Read the model definition and answer for the solid it produces. Units are mm, in the model's axes. Face numbers are marked on the shaded views. A direction names the side the tool comes from. Coordinates: 2 decimals unless noted, no trailing zeros. Write each loop counter-clockwise with the first axis right and the second up, starting at its lowest first coordinate (ties: lowest second). Pieces come first, ordered by that corner, then holes.
1) The part is cut by section B-B (x = 181.5). Determine the outline of the cut face in (y, z), then the cut area to 3 significant figures.
2) Which of the six approach directions +Z, -Z, +X, -X, +Y, -Y give full straight-line access (tool end or side, diameter ignored) to the marked faces 1, 2 and 3?
3) Find the intervals of material crossed by line 1 (Y direction, x = 63.5, z = 29); line 2 (X direction, y = 35, z = 9); line 3 (X direction, y = -31, z = -28.5), in increasing order.
4) The part is cut by section A-A (x = 71). Determine the outline of the cut face in (y, z), then the cut area to 3 significant figures.
5) Determine the mould class of the marked faces 4, 5 and 6 for opening direction X: +X half, -X half, draft (parallel to the pull), parting line (faces both ways), or undercut.
6) Each of these flat-tipped pins is pushed along its axis until it touches: pin 1 Ø2 at (x, y) = (318.5, -4.5) entering from -Z; pin 2 Ø1.5 at (x, z) = (123, -9.5) entering from +Y; pin 3 Ø5.5 at (x, y) = (256.5, -12.5) entering from -Z. Where does it stop, or does it pass through?
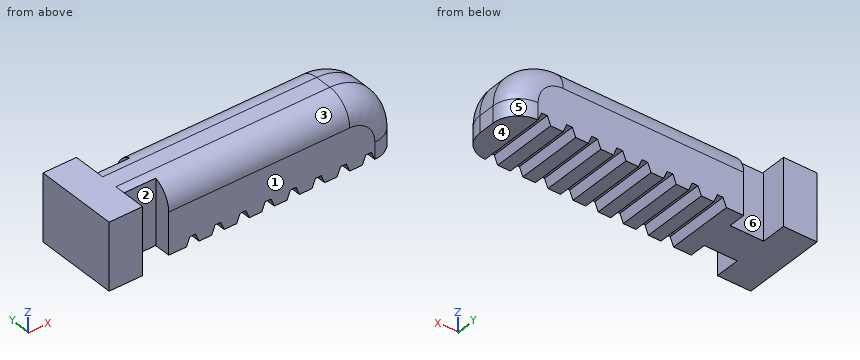
from build123d import *

# Parameters (mm, degrees)
BOSS_EXTRUDE1_DEPTH          = 40
FILLET1_R                    = 60
FILLET2_R                    = 30
SKETCH3_W                    = 15
SKETCH3_H                    = 109.922704731
CUT_EXTRUDE1_DEPTH           = 10
CUT_EXTRUDE1_DRAFT           = -22
CUT_EXTRUDE1_PROFILE_2_DEPTH = 10
CUT_EXTRUDE1_PROFILE_2_DRAFT = -22
CUT_EXTRUDE1_PROFILE_3_DEPTH = 10
CUT_EXTRUDE1_PROFILE_3_DRAFT = -22
CUT_EXTRUDE1_PROFILE_4_DEPTH = 10
CUT_EXTRUDE1_PROFILE_4_DRAFT = -22
CUT_EXTRUDE1_PROFILE_5_DEPTH = 10
CUT_EXTRUDE1_PROFILE_5_DRAFT = -22
CUT_EXTRUDE1_PROFILE_6_DEPTH = 10
CUT_EXTRUDE1_PROFILE_6_DRAFT = -22
CUT_EXTRUDE1_PROFILE_7_DEPTH = 10
CUT_EXTRUDE1_PROFILE_7_DRAFT = -22
CUT_EXTRUDE1_PROFILE_8_DEPTH = 10
CUT_EXTRUDE1_PROFILE_8_DRAFT = -22


with BuildPart() as part:
    # Sketch1 → Boss-Extrude1 (new, symmetric)
    with BuildSketch(Plane.XY):
        Polygon((0, 41.520471033), (0, -58.474576271), (40, -58.474576271), (40, -28.474576271), (79.370562847, -28.474576271), (79.370562847, -48.090018927), (355.561633386, -48.090018927), (355.561633386, -28.474576271), (355.561633386, 11.525423729), (355.561633386, 31.909981073), (80, 31.909981073), (80, 11.520471033), (40, 11.520471033), (40, 41.520471033), align=None)
    extrude(amount=BOSS_EXTRUDE1_DEPTH, both=True)

    # Fillet1
    fillet1_edges = [part.edges().sort_by_distance(p)[0] for p in [
        (355.561633386, -8.090018927, 40),
    ]]
    fillet(fillet1_edges, radius=FILLET1_R)

    # Fillet2
    # the kernel refuses this fillet: 30 mm, written as the material it takes off along each edge
    with BuildSketch(Plane(origin=(355.561633386, -48.090018927, -115), x_dir=(0, 1, 0), z_dir=(0, 0, 1)), Plane(origin=(355.561633386, 31.909981073, -115), x_dir=(-1, 0, 0), z_dir=(0, 0, 1))) as fillet2_piece_1:
        with BuildLine():
            CenterArc((FILLET2_R, FILLET2_R), FILLET2_R, 180, 90)
            Line((0, FILLET2_R), (0, 0))
            Line((0, 0), (FILLET2_R, 0))
        make_face()
    extrude(amount=95, mode=Mode.SUBTRACT)
    with BuildSketch(Plane(origin=(295.561633386, -48.090018927, -20), x_dir=(1, 0, 0), z_dir=(0, 0, -1))) as fillet2_piece_2:
        with BuildLine():
            CenterArc((60 - FILLET2_R, -FILLET2_R), FILLET2_R, 0, 90)
            Line((60 - FILLET2_R, 0), (60, 0))
            Line((60, 0), (60, -FILLET2_R))
        make_face()
    revolve(axis=Axis((295.561633386, -48.090018927, -20), (0, -1, 0)), revolution_arc=90, mode=Mode.SUBTRACT)
    with BuildSketch(Plane(origin=(295.561633386, 31.909981073, -20), x_dir=(1, 0, 0), z_dir=(0, 0, -1))) as fillet2_piece_3:
        with BuildLine():
            CenterArc((60 - FILLET2_R, FILLET2_R), FILLET2_R, 270, 90)
            Line((60, FILLET2_R), (60, 0))
            Line((60, 0), (60 - FILLET2_R, 0))
        make_face()
    revolve(axis=Axis((295.561633386, 31.909981073, -20), (0, -1, 0)), revolution_arc=90, mode=Mode.SUBTRACT)
    with BuildSketch(Plane(origin=(4.370562847, -48.090018927, 40), x_dir=(0, 1, 0), z_dir=(1, 0, 0))) as fillet2_piece_4_section:
        with BuildLine():
            CenterArc((FILLET2_R, -FILLET2_R), FILLET2_R, 90, 90)
            Line((0, -FILLET2_R), (0, 0))
            Line((0, 0), (FILLET2_R, 0))
        make_face()
    fillet2_piece_4 = extrude(amount=291.191070539, mode=Mode.PRIVATE)
    fillet2_piece_4 = split(fillet2_piece_4, bisect_by=Plane(origin=(40, -25.894757841, 39.446684124), z_dir=(1, 0, 0)), keep=Keep.TOP, mode=Mode.PRIVATE)
    add(fillet2_piece_4, mode=Mode.SUBTRACT)
    with BuildSketch(Plane(origin=(295.561633386, 31.909981073, 40), x_dir=(0, 0, -1), z_dir=(-1, 0, 0))) as fillet2_piece_5_section:
        with BuildLine():
            CenterArc((FILLET2_R, FILLET2_R), FILLET2_R, 180, 90)
            Line((0, FILLET2_R), (0, 0))
            Line((0, 0), (FILLET2_R, 0))
        make_face()
    fillet2_piece_5 = extrude(amount=290.561633386, mode=Mode.PRIVATE)
    fillet2_piece_5 = split(fillet2_piece_5, bisect_by=Plane(origin=(40, 26.935715602, 30.794780606), z_dir=(1, 0, 0)), keep=Keep.TOP, mode=Mode.PRIVATE)
    add(fillet2_piece_5, mode=Mode.SUBTRACT)


with BuildPart() as cut_extrude1_tool:
    # Sketch3 → Cut-Extrude1 (with draft: the straight prism first)
    with BuildSketch(Plane(origin=(0, 0, -40), x_dir=(-1, 0, 0), z_dir=(0, 0, -1))):
        with Locations((-318.061633386, -9.051561529)):
            Rectangle(SKETCH3_W, SKETCH3_H)
    extrude(amount=-CUT_EXTRUDE1_DEPTH)
    # Cut-Extrude1: the draft: its side faces are tilted about the plane it starts from
    cut_extrude1_sides = [cut_extrude1_tool.faces().sort_by_distance(p)[0] for p in [
        (325.561633386, -9.051561529, -35),
        (318.061633386, -64.012913894, -35),
        (310.561633386, -9.051561529, -35),
        (318.061633386, 45.909790837, -35),
    ]]
    draft(cut_extrude1_sides, Plane(origin=(0, 0, -40), x_dir=(-1, 0, 0), z_dir=(0, 0, -1)), CUT_EXTRUDE1_DRAFT)


with BuildPart() as part_1:
    add(part.part)

    # Cut-Extrude1: cut by cut_extrude1_tool
    add(cut_extrude1_tool.part, mode=Mode.SUBTRACT)


with BuildPart() as cut_extrude1_profile_2_tool:
    # Sketch3 → Cut-Extrude1 profile 2 (with draft: the straight prism first)
    with BuildSketch(Plane(origin=(0, 0, -40), x_dir=(-1, 0, 0), z_dir=(0, 0, -1))):
        with Locations((-288.061633386, -9.051561529)):
            Rectangle(SKETCH3_W, SKETCH3_H)
    extrude(amount=-CUT_EXTRUDE1_PROFILE_2_DEPTH)
    # Cut-Extrude1 profile 2: the draft: its side faces are tilted about the plane it starts from
    cut_extrude1_profile_2_sides = [cut_extrude1_profile_2_tool.faces().sort_by_distance(p)[0] for p in [
        (295.561633386, -9.051561529, -35),
        (288.061633386, -64.012913894, -35),
        (280.561633386, -9.051561529, -35),
        (288.061633386, 45.909790837, -35),
    ]]
    draft(cut_extrude1_profile_2_sides, Plane(origin=(0, 0, -40), x_dir=(-1, 0, 0), z_dir=(0, 0, -1)), CUT_EXTRUDE1_PROFILE_2_DRAFT)


with BuildPart() as part_2:
    add(part_1.part)

    # Cut-Extrude1 profile 2: cut by cut_extrude1_profile_2_tool
    add(cut_extrude1_profile_2_tool.part, mode=Mode.SUBTRACT)


with BuildPart() as cut_extrude1_profile_3_tool:
    # Sketch3 → Cut-Extrude1 profile 3 (with draft: the straight prism first)
    with BuildSketch(Plane(origin=(0, 0, -40), x_dir=(-1, 0, 0), z_dir=(0, 0, -1))):
        with Locations((-258.061633386, -9.051561529)):
            Rectangle(SKETCH3_W, SKETCH3_H)
    extrude(amount=-CUT_EXTRUDE1_PROFILE_3_DEPTH)
    # Cut-Extrude1 profile 3: the draft: its side faces are tilted about the plane it starts from
    cut_extrude1_profile_3_sides = [cut_extrude1_profile_3_tool.faces().sort_by_distance(p)[0] for p in [
        (265.561633386, -9.051561529, -35),
        (258.061633386, -64.012913894, -35),
        (250.561633386, -9.051561529, -35),
        (258.061633386, 45.909790837, -35),
    ]]
    draft(cut_extrude1_profile_3_sides, Plane(origin=(0, 0, -40), x_dir=(-1, 0, 0), z_dir=(0, 0, -1)), CUT_EXTRUDE1_PROFILE_3_DRAFT)


with BuildPart() as part_3:
    add(part_2.part)

    # Cut-Extrude1 profile 3: cut by cut_extrude1_profile_3_tool
    add(cut_extrude1_profile_3_tool.part, mode=Mode.SUBTRACT)


with BuildPart() as cut_extrude1_profile_4_tool:
    # Sketch3 → Cut-Extrude1 profile 4 (with draft: the straight prism first)
    with BuildSketch(Plane(origin=(0, 0, -40), x_dir=(-1, 0, 0), z_dir=(0, 0, -1))):
        with Locations((-228.061633386, -9.051561529)):
            Rectangle(SKETCH3_W, SKETCH3_H)
    extrude(amount=-CUT_EXTRUDE1_PROFILE_4_DEPTH)
    # Cut-Extrude1 profile 4: the draft: its side faces are tilted about the plane it starts from
    cut_extrude1_profile_4_sides = [cut_extrude1_profile_4_tool.faces().sort_by_distance(p)[0] for p in [
        (235.561633386, -9.051561529, -35),
        (228.061633386, -64.012913894, -35),
        (220.561633386, -9.051561529, -35),
        (228.061633386, 45.909790837, -35),
    ]]
    draft(cut_extrude1_profile_4_sides, Plane(origin=(0, 0, -40), x_dir=(-1, 0, 0), z_dir=(0, 0, -1)), CUT_EXTRUDE1_PROFILE_4_DRAFT)


with BuildPart() as part_4:
    add(part_3.part)

    # Cut-Extrude1 profile 4: cut by cut_extrude1_profile_4_tool
    add(cut_extrude1_profile_4_tool.part, mode=Mode.SUBTRACT)


with BuildPart() as cut_extrude1_profile_5_tool:
    # Sketch3 → Cut-Extrude1 profile 5 (with draft: the straight prism first)
    with BuildSketch(Plane(origin=(0, 0, -40), x_dir=(-1, 0, 0), z_dir=(0, 0, -1))):
        with Locations((-198.061633386, -9.051561529)):
            Rectangle(SKETCH3_W, SKETCH3_H)
    extrude(amount=-CUT_EXTRUDE1_PROFILE_5_DEPTH)
    # Cut-Extrude1 profile 5: the draft: its side faces are tilted about the plane it starts from
    cut_extrude1_profile_5_sides = [cut_extrude1_profile_5_tool.faces().sort_by_distance(p)[0] for p in [
        (205.561633386, -9.051561529, -35),
        (198.061633386, -64.012913894, -35),
        (190.561633386, -9.051561529, -35),
        (198.061633386, 45.909790837, -35),
    ]]
    draft(cut_extrude1_profile_5_sides, Plane(origin=(0, 0, -40), x_dir=(-1, 0, 0), z_dir=(0, 0, -1)), CUT_EXTRUDE1_PROFILE_5_DRAFT)


with BuildPart() as part_5:
    add(part_4.part)

    # Cut-Extrude1 profile 5: cut by cut_extrude1_profile_5_tool
    add(cut_extrude1_profile_5_tool.part, mode=Mode.SUBTRACT)


with BuildPart() as cut_extrude1_profile_6_tool:
    # Sketch3 → Cut-Extrude1 profile 6 (with draft: the straight prism first)
    with BuildSketch(Plane(origin=(0, 0, -40), x_dir=(-1, 0, 0), z_dir=(0, 0, -1))):
        with Locations((-168.061633386, -9.051561529)):
            Rectangle(SKETCH3_W, SKETCH3_H)
    extrude(amount=-CUT_EXTRUDE1_PROFILE_6_DEPTH)
    # Cut-Extrude1 profile 6: the draft: its side faces are tilted about the plane it starts from
    cut_extrude1_profile_6_sides = [cut_extrude1_profile_6_tool.faces().sort_by_distance(p)[0] for p in [
        (175.561633386, -9.051561529, -35),
        (168.061633386, -64.012913894, -35),
        (160.561633386, -9.051561529, -35),
        (168.061633386, 45.909790837, -35),
    ]]
    draft(cut_extrude1_profile_6_sides, Plane(origin=(0, 0, -40), x_dir=(-1, 0, 0), z_dir=(0, 0, -1)), CUT_EXTRUDE1_PROFILE_6_DRAFT)


with BuildPart() as part_6:
    add(part_5.part)

    # Cut-Extrude1 profile 6: cut by cut_extrude1_profile_6_tool
    add(cut_extrude1_profile_6_tool.part, mode=Mode.SUBTRACT)


with BuildPart() as cut_extrude1_profile_7_tool:
    # Sketch3 → Cut-Extrude1 profile 7 (with draft: the straight prism first)
    with BuildSketch(Plane(origin=(0, 0, -40), x_dir=(-1, 0, 0), z_dir=(0, 0, -1))):
        with Locations((-138.061633386, -9.051561529)):
            Rectangle(SKETCH3_W, SKETCH3_H)
    extrude(amount=-CUT_EXTRUDE1_PROFILE_7_DEPTH)
    # Cut-Extrude1 profile 7: the draft: its side faces are tilted about the plane it starts from
    cut_extrude1_profile_7_sides = [cut_extrude1_profile_7_tool.faces().sort_by_distance(p)[0] for p in [
        (145.561633386, -9.051561529, -35),
        (138.061633386, -64.012913894, -35),
        (130.561633386, -9.051561529, -35),
        (138.061633386, 45.909790837, -35),
    ]]
    draft(cut_extrude1_profile_7_sides, Plane(origin=(0, 0, -40), x_dir=(-1, 0, 0), z_dir=(0, 0, -1)), CUT_EXTRUDE1_PROFILE_7_DRAFT)


with BuildPart() as part_7:
    add(part_6.part)

    # Cut-Extrude1 profile 7: cut by cut_extrude1_profile_7_tool
    add(cut_extrude1_profile_7_tool.part, mode=Mode.SUBTRACT)


with BuildPart() as cut_extrude1_profile_8_tool:
    # Sketch3 → Cut-Extrude1 profile 8 (with draft: the straight prism first)
    with BuildSketch(Plane(origin=(0, 0, -40), x_dir=(-1, 0, 0), z_dir=(0, 0, -1))):
        with Locations((-108.061633386, -9.051561529)):
            Rectangle(SKETCH3_W, SKETCH3_H)
    extrude(amount=-CUT_EXTRUDE1_PROFILE_8_DEPTH)
    # Cut-Extrude1 profile 8: the draft: its side faces are tilted about the plane it starts from
    cut_extrude1_profile_8_sides = [cut_extrude1_profile_8_tool.faces().sort_by_distance(p)[0] for p in [
        (115.561633386, -9.051561529, -35),
        (108.061633386, -64.012913894, -35),
        (100.561633386, -9.051561529, -35),
        (108.061633386, 45.909790837, -35),
    ]]
    draft(cut_extrude1_profile_8_sides, Plane(origin=(0, 0, -40), x_dir=(-1, 0, 0), z_dir=(0, 0, -1)), CUT_EXTRUDE1_PROFILE_8_DRAFT)


with BuildPart() as part_8:
    add(part_7.part)

    # Cut-Extrude1 profile 8: cut by cut_extrude1_profile_8_tool
    add(cut_extrude1_profile_8_tool.part, mode=Mode.SUBTRACT)


solid = part_8.part
Reported:
1. outline: (-48.09, -40) - (31.91, -40) - (31.91, 10) arc R30 ccw to (1.91, 40) - (-18.09, 40) arc R30 ccw to (-48.09, 10) - close
1. area: 6,010 mm2
2. face 1: +Z, -Z, +X, -Y
2. face 2: +Z, -Z, -Y
2. face 3: +Z, +X, -Y
3. line 1: y = -28.47 to 11.52
3. line 2: x = 0 to 40
3. line 3: x = 0 to 40, 79.37 to 352.64
4. outline: (-28.47, -40) - (11.52, -40) - (11.52, 38.42) arc R30 ccw to (1.91, 40) - (-18.09, 40) arc R30 ccw to (-28.47, 38.15) - close
4. area: 3,190 mm2
5. face 4: draft
5. face 5: +X half
5. face 6: undercut
6. pin 1: stops at z = -30
6. pin 2: stops at y = 31.91
6. pin 3: stops at z = -32.11
